Read the model definition and answer for the solid it produces. Units are mm, in the model's axes. A direction names the side the tool comes from. Coordinates: 2 decimals unless noted, no trailing zeros. Write each loop counter-clockwise with the first axis right and the second up, starting at its lowest first coordinate (ties: lowest second). Pieces come first, ordered by that corner, then holes. Notation, with made-up numbers: (47.25, -38) -> (56.25, -38) arc R33 cw to (56.25, 0) -> close; hole circle Ø8 at (47.5, 71.25). An arc over 180 degrees is marked (long way). Answer as a JSON object with one key per item and string values. Group by question number.
(1) Find section B-B (x = 37.5). Give the vertices of the cut face in (y, z).
(2) For a pull along X with two mould halves and no side action, classify faces 1 (the face through (74.764, -10, 11)), 2 (the face through (39, -10, 16.564)), 3 (the face through (80, -13, 10)), 4 (the face through (39, -25.4, 10)) as +X half, -X half, draft (parallel to the pull), parting line (faces both ways), or undercut.
(3) Which of the six approach directions +Z, -Z, +X, -X, +Y, -Y give full straight-line access (tool end or side, diameter ignored) to faces 5 (the face through (39, -20, 12)), 6 (the face through (39, -13, 0))?
(4) Flat-ended cylindrical pins translate along their axes: P1, Ø2, axis at x = 36, z = 18, coming from the +Y side; P2, Ø6, axis at x = 66.5, z = 13.5, coming from the +Y side. Find the tip coordinate at first contact, or state that the pin passes through.
(5) Straight lines are drawn through the part: L1, parallel to X at y = -10.75, z = 12; L2, parallel to Z at x = 15, y = -16.5; L3, parallel to Y at x = 13, z = 10. For each, find the intervals that lie inside material, in ascending order.
(6) Find section C-C (z = 12.5). Give the vertices of the cut face in (x, y).
(7) Find section A-A (y = -2.5). Give the vertices of the cut face in (x, z).
from build123d import *

# Parameters (mm, degrees)
F0_W     = 80
F0_H     = 20
F1_DEPTH = 25.4
F2_W     = 70
F2_H     = 10
F3_DEPTH = 20
F4_DEPTH = 20


with BuildPart() as f1:
    # F0 (on Front) → F1 (new body)
    with BuildSketch(Plane.XZ):
        with Locations((40, 10)):
            Rectangle(F0_W, F0_H)
    extrude(amount=F1_DEPTH)

    # F2 (on Front) → F3 (cut)
    with BuildSketch(Plane.XZ):
        with Locations((39.764389, 11.563558)):
            Rectangle(F2_W, F2_H)
    extrude(amount=-F3_DEPTH, mode=Mode.SUBTRACT)

    # F2 (on Front) → F4 (cut)
    with BuildSketch(Plane.XZ):
        with Locations((39.764389, 11.563558)):
            Rectangle(F2_W, F2_H)
    extrude(amount=F4_DEPTH, mode=Mode.SUBTRACT)


solid = f1.part
Results below:
{
 "1": {"outline": "(-25.4, 0) -> (0, 0) -> (0, 6.56) -> (-20, 6.56) -> (-20, 16.56) -> (0, 16.56) -> (0, 20) -> (-25.4, 20) -> close"},
 "2": {"face 1": "undercut", "face 2": "undercut", "face 3": "+X half", "face 4": "draft"},
 "3": {"face 5": "+Y", "face 6": "-Z, +X, -X, +Y, -Y"},
 "4": {"P1": "stops at y = 0", "P2": "stops at y = -20"},
 "5": {"L1": "x = 0 to 4.76, 74.76 to 80", "L2": "z = 0 to 6.56, 16.56 to 20", "L3": "y = -25.4 to -20"},
 "6": {"outline": "(0, -25.4) -> (80, -25.4) -> (80, 0) -> (74.76, 0) -> (74.76, -20) -> (4.76, -20) -> (4.76, 0) -> (0, 0) -> close"},
 "7": {"outline": "(0, 0) -> (80, 0) -> (80, 20) -> (0, 20) -> close; hole (4.76, 6.56) -> (74.76, 6.56) -> (74.76, 16.56) -> (4.76, 16.56) -> close"}
}
